```python
from build123d import *

# Parameters (mm, degrees)
F0_W     = 101.6
F0_H     = 101.6
F0_R     = 44.45
F1_DEPTH = 22.86
F3_R     = 1.905
F4_DEPTH = 101.601
F2_R     = 1.905
F5_DEPTH = 6.3918402903
F6_W     = 101.6
F6_H     = 101.6
F7_DEPTH = 2.54
F8_R     = 47.625
F9_DEPTH = 3.175


with BuildPart() as f1:
    # F0 (on Front) → F1 (new body)
    with BuildSketch(Plane.XZ):
        Rectangle(F0_W, F0_H)
        Circle(F0_R, mode=Mode.SUBTRACT)
    extrude(amount=F1_DEPTH)

    # F3 (on face) → F4 (cut, through all)
    with BuildSketch(Plane.YZ.offset(50.8)):
        with Locations((-11.43, 0)):
            Circle(F3_R)
    extrude(amount=-F4_DEPTH, mode=Mode.SUBTRACT)

    # F2 (on face) → F5 (cut, through all)
    with BuildSketch(Plane(origin=(0, 0, -50.8), x_dir=(1, 0, 0), z_dir=(0, 0, -1))):
        with Locations((0, 11.43)):
            Circle(F2_R)
    extrude(amount=-F5_DEPTH, mode=Mode.SUBTRACT)

    # F6 (on Front) → F7 (join)
    with BuildSketch(Plane.XZ):
        Rectangle(F6_W, F6_H)
    extrude(amount=-F7_DEPTH)

    # F8 (on face) → F9 (cut)
    with BuildSketch(Plane.XZ.offset(22.86)):
        Circle(F8_R)
    extrude(amount=-F9_DEPTH, mode=Mode.SUBTRACT)


solid = f1.part
```
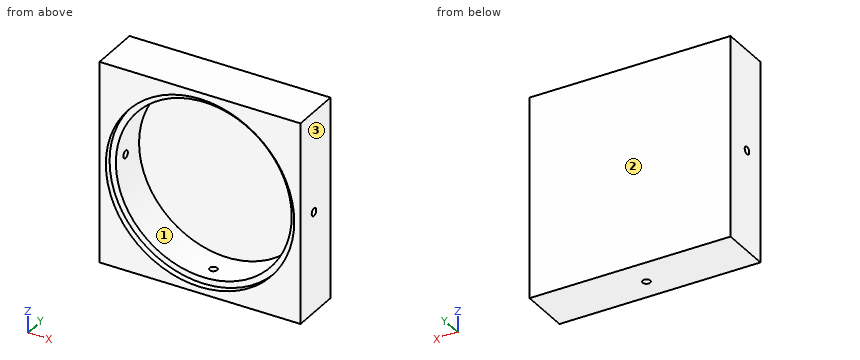
Here's how the part is built. I have some questions about the finished solid (model axes, mm). Face numbers are marked on the shaded views. Give positions to 0.01 mm unless a question says otherwise; leave off trailing zeros. Loops run counter-clockwise (first coordinate to the right, second up) from the corner with the lowest first, then second, coordinate; pieces in that order, holes last. Notation, with made-up numbers: (-36.5, -27.5) -> (-20.5, -27.5) arc R12 cw to (-20.5, -22.5) -> close; hole circle Ø3 at (62, 2.25). An arc over 180 degrees is marked (long way). Use one line per item in the form item = value. Start each with the question number.
1) Thinking about a two-plate mould opening in X: for the marked faces 1, 2 and 3, which applies, +X half, -X half, draft (parallel to the pull), parting line (faces both ways), or undercut?
2) Imagine slicing it at A-A (z = 0). Please give me the cut outline in (x, y) (3 decimals).
3) Imagine slicing it at D-D (x = 16). Please give me the cut outline in (y, z) (1 decimal).
4) Imagine slicing it at C-C (y = -11.43). Please give me the cut outline in (x, z) (3 decimals), then the cut area to 3 significant figures.
5) Please list where these lines run through material, in increasing order: line 1 along Z through (x, y) = (48.75, -11.43) (3 decimals); line 2 along Y through (x, z) = (-10, 2.5); line 3 along Z through (x, y) = (13, -18.5).
6) Imagine slicing it at B-B (x = 0). Please give me the cut outline in (y, z) (3 decimals), then the cut area to 3 significant figures.
7) For P1, Ø6, axis at y = -11.43, z = 0, coming from the +X side; P2, Ø6, axis at x = -14.5, z = 8.5, coming from the -Y side, each with a flat end and sliding along its axis, tell me the tip position at first contact or that it passes through.
Check values:
q1.face_1 = undercut
q1.face_2 = draft
q1.face_3 = +X half
q2.outline = (-50.8, -22.86) -> (-47.625, -22.86) -> (-47.625, -19.685) -> (-44.45, -19.685) -> (-44.45, -13.335) -> (-50.8, -13.335) -> close; (-50.8, -9.525) -> (-44.45, -9.525) -> (-44.45, 0) -> (44.45, 0) -> (44.45, -9.525) -> (50.8, -9.525) -> (50.8, 2.54) -> (-50.8, 2.54) -> close; (44.45, -19.685) -> (47.625, -19.685) -> (47.625, -22.86) -> (50.8, -22.86) -> (50.8, -13.335) -> (44.45, -13.335) -> close
q3.outline = (-22.9, -50.8) -> (2.5, -50.8) -> (2.5, 50.8) -> (-22.9, 50.8) -> (-22.9, 44.9) -> (-19.7, 44.9) -> (-19.7, 41.5) -> (0, 41.5) -> (0, -41.5) -> (-19.7, -41.5) -> (-19.7, -44.9) -> (-22.9, -44.9) -> close
q4.outline = (-50.8, -50.8) -> (-1.905, -50.8) -> (-1.905, -44.409) arc R44.45 cw to (-44.409, -1.905) -> (-50.8, -1.905) -> close; (-50.8, 1.905) -> (-44.409, 1.905) arc R44.45 cw to (44.409, 1.905) -> (50.8, 1.905) -> (50.8, 50.8) -> (-50.8, 50.8) -> close; (1.905, -50.8) -> (50.8, -50.8) -> (50.8, -1.905) -> (44.409, -1.905) arc R44.45 cw to (1.905, -44.409) -> close
q4.area = 4,040 mm^2
q5.line_1 = -50.8 to -1.905, 1.905 to 50.8
q5.line_2 = 0 to 2.54
q5.line_3 = -50.8 to -42.51, 42.51 to 50.8
q6.outline = (-22.86, -50.8) -> (-13.335, -50.8) -> (-13.335, -44.45) -> (-19.685, -44.45) -> (-19.685, -47.625) -> (-22.86, -47.625) -> close; (-22.86, 47.625) -> (-19.685, 47.625) -> (-19.685, 44.45) -> (0, 44.45) -> (0, -44.45) -> (-9.525, -44.45) -> (-9.525, -50.8) -> (2.54, -50.8) -> (2.54, 50.8) -> (-22.86, 50.8) -> close
q6.area = 504 mm^2
q7.P1 = 50.8
q7.P2 = 0
